Can you work these out from the drawing? Everything is in mm from the part's minimum corner. Round coordinates to 2 decimals unless told otherwise and drop trailing zeros. Write each loop counter-clockwise with the first axis right and the second up, starting at its lowest first coordinate (ties: lowest second). Pieces come first, ordered by that corner, then holes. Notation, with made-up numbers: M 61.5,84 L 90.5,84 A23 ccw 90.5,98 Z; hole C 2,89.5 d9. An arc over 180 degrees is marked long. Use a Markdown table: item, result. Add a question column.
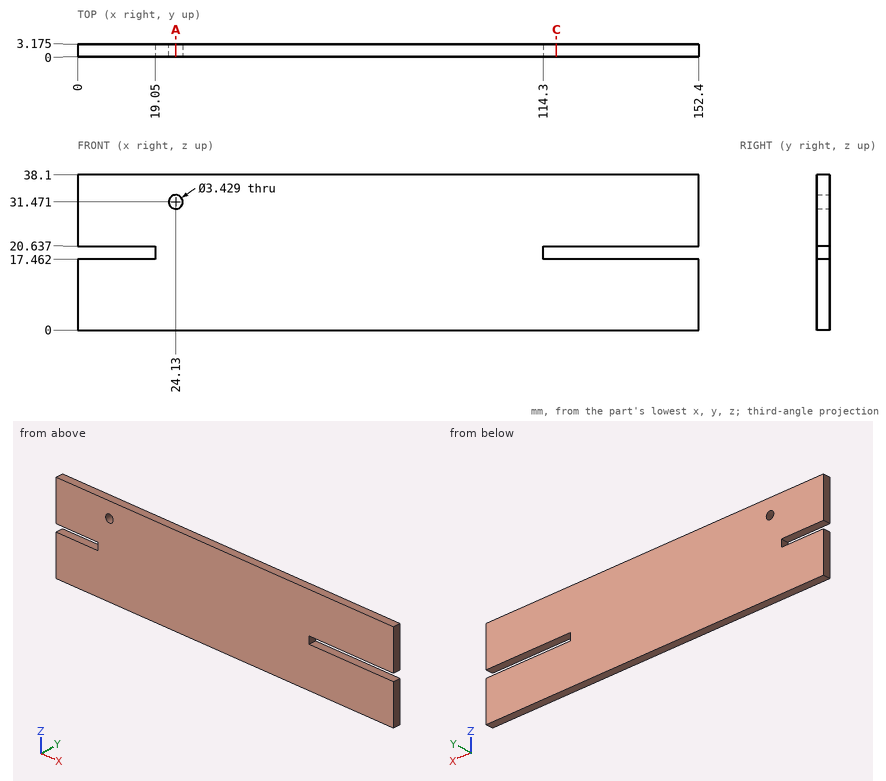
Item 1: Imagine slicing it at A-A on x = 24.13. List the corners of the cut face in (y, z) for me (1 decimal).
Item 2: Imagine slicing it at C-C on x = 117.5. List the corners of the cut face in (y, z) for me (1 decimal), plus the area to 3 significant figures.
Item 3: For pin 1 Ø1.6 at (x, y) = (6.5, 2) entering from -Z, with a flat end and sliding along its axis, tell me the tip position at first contact or that it passes through.
Item 4: I need wall thicknesses on probe 1 along Z at (x, y) = (24.13, 1.15) (1 decimal); probe 2 along Z at (x, y) = (144, 1.65). Which ranges of each line are inside material? Lowest first, please. Write a range as from..to.
The answers:
| question | item | result |
|---|---|---|
| 1 | outline | M 0,0 L 3.2,0 L 3.2,29.8 L 0,29.8 Z; M 0,33.2 L 3.2,33.2 L 3.2,38.1 L 0,38.1 Z |
| 2 | outline | M 0,0 L 3.2,0 L 3.2,17.5 L 0,17.5 Z; M 0,20.6 L 3.2,20.6 L 3.2,38.1 L 0,38.1 Z |
| 2 | area | 111 mm² |
| 3 | pin 1 | z = 0 |
| 4 | probe 1 | 0..29.8, 33.2..38.1 |
| 4 | probe 2 | 0..17.46, 20.64..38.1 |
